Check sheet for the modelled part. Datum: model origin and axes. Units: mm. A direction names the side the tool comes from. Round coordinates to 2 decimals unless told otherwise and drop trailing zeros. Order: outer loops, then holes, each group sorted by start corner. A loop starts at its lowest first (then second) coordinate and runs counter-clockwise, first axis right, second up. Notation, with made-up numbers: M -4,52 L 10,52 A31 ccw 10,80 Z; hole C -32,15.5 d1. An arc over 180 degrees is marked long. One line per item, written item: value. Start each with the question number.
(1) Cross-section at C-C, the plane y = 3. Enter the section's corners in (x, z).
(2) Access from +Z, -Z, +X, -X, +Y, -Y to the whole of each face (thin tool, end or side, straight path). Record for faces 5 (the face through (-0.97, 20.73, -1.27)), 6 (the face through (1, 40, 0)), 7 (the face through (-2.44, 0.99, -0.54)).
(3) Depth check by flat-ended pin: pin 1 Ø2 at (y, z) = (37, 0) entering from -X; pin 2 Ø2 at (x, z) = (1.5, -1.5) entering from +Y. Enter the tip coordinate at first touch or a pass-through.
(4) Release check for a two-part mould opening along Y. For faces 1 (the face through (0, 0, 0)), 2 (the face through (-0.506, 41.014, -0.323)), 3 (the face through (1, 42, 0)), 4 (the face through (-2, 2, 0)) record: released by +Y, released by -Y, zero draft, split by the parting line, or undercut.
(5) Cross-section at A-A, the plane x = 0. Enter the section's corners in (y, z), and give its area (3 significant figures).
(6) Thickness scan on L1, parallel to Y at x = 1.35, z = -0.2; L2, parallel to Y at x = -1.2, z = 2.1; L3, parallel to X at y = 13, z = -1.35. Record the ranges inside material, lowest first.
(7) Cross-section at B-B, the plane z = -1.1. Enter the section's corners in (x, y) (3 decimals), and give its area (3 significant figures).
(8) Cross-section at D-D, the plane x = -2.1. Enter the section's corners in (y, z), and give its area (3 significant figures).
from build123d import *

# Parameters (mm, degrees)
SKETCH1_R           = 1.6
BOSS_EXTRUDE1_DEPTH = 43
SKETCH2_W           = 1
SKETCH2_H           = 2
SKETCH3_R           = 2.5
BOSS_EXTRUDE2_DEPTH = 2


with BuildPart() as part:
    # Sketch1 → Boss-Extrude1 (new body)
    with BuildSketch(Plane(origin=(0, 0, 0), x_dir=(1, 0, 0), z_dir=(0, 1, 0))):
        with Locations(Location((0, 0, 0), (0, 0, 270))):
            Circle(SKETCH1_R)
    extrude(amount=BOSS_EXTRUDE1_DEPTH)

    # Sketch2 → Cut-Revolve1 (revolve, cut)
    with BuildSketch(Plane.XY, mode=Mode.PRIVATE) as cut_revolve1_sk:
        with Locations((1.1, 41)):
            Rectangle(SKETCH2_W, SKETCH2_H)
    revolve(cut_revolve1_sk.sketch.rotate(Axis((0, 0, 0), (0, 1, 0)), 90), axis=Axis((0, 0, 0), (0, 1, 0)), mode=Mode.SUBTRACT)

    # Sketch3 → Boss-Extrude2 (add)
    with BuildSketch(Plane(origin=(0, 0, 0), x_dir=(1, 0, 0), z_dir=(0, 1, 0))):
        with Locations(Location((0, 0, 0), (0, 0, 270))):
            Circle(SKETCH3_R)
    extrude(amount=BOSS_EXTRUDE2_DEPTH)


solid = part.part
Values found:
1. outline: C 0,0 d3.2
2. face 5: +Y
2. face 6: none
2. face 7: +Y, -Y
3. pin 1: x = -1.6
3. pin 2: y = 43
4. face 1: released by -Y
4. face 2: undercut
4. face 3: undercut
4. face 4: released by +Y
5. outline: M 0,-2.5 L 2,-2.5 L 2,-1.6 L 40,-1.6 L 40,-0.6 L 42,-0.6 L 42,-1.6 L 43,-1.6 L 43,1.6 L 42,1.6 L 42,0.6 L 40,0.6 L 40,1.6 L 2,1.6 L 2,2.5 L 0,2.5 Z
5. area: 137 mm^2
6. L1: 0 to 40, 42 to 43
6. L2: 0 to 2
6. L3: -0.86 to 0.86
7. outline: M -2.245,0 L 2.245,0 L 2.245,2 L 1.162,2 L 1.162,40 L -1.162,40 L -1.162,2 L -2.245,2 Z; M -1.162,42 L 1.162,42 L 1.162,43 L -1.162,43 Z
7. area: 99.6 mm^2
8. outline: M 0,-1.36 L 2,-1.36 L 2,1.36 L 0,1.36 Z
8. area: 5.43 mm^2
